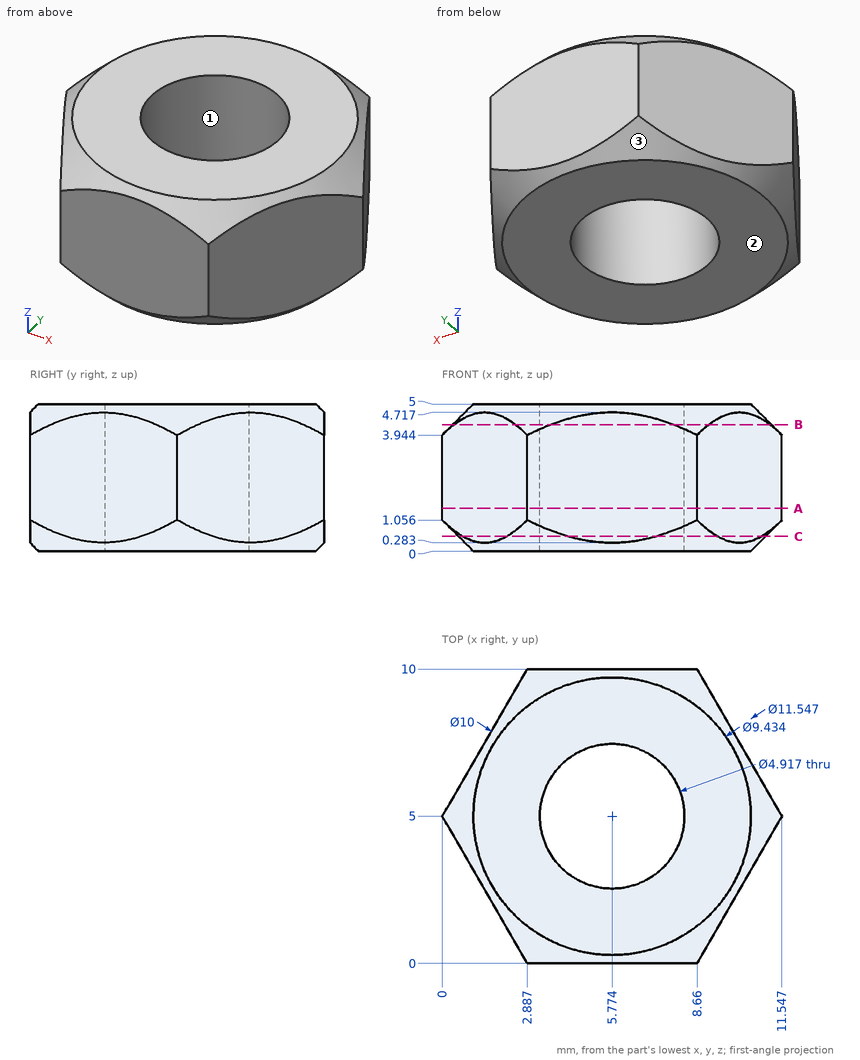
Verification items for this drawing (mm, ordinates from the low corner). Give positions to 0.01 mm unless a question says otherwise; leave off trailing zeros. Write each loop counter-clockwise with the first axis right and the second up, starting at its lowest first coordinate (ties: lowest second). Pieces come first, ordered by that corner, then holes.
1) Section check A-A, the plane z = 1.45. Record the boundary of the cut face in (x, y).
2) Section check B-B, the plane z = 4.3. Record the boundary of the cut face in (x, y) (1 decimal).
3) Section check C-C, the plane z = 0.5. Record the boundary of the cut face in (x, y) (1 decimal).
4) Material ranges on L1, parallel to Y at x = 8, z = 0.55 (1 decimal); L2, parallel to Y at x = 5.25, z = 2.7; L3, parallel to X at y = 1.5, z = 3.25 (1 decimal), recorded low to high.
5) Gauge pin test, flat ends, axial feed: pin 1 (3 mm diameter, centred on y = 1.5, z = 2.5, fed in from +X); pin 2 (2 mm diameter, centred on x = 7, y = 4.5, fed in from -Z). Record the tip position at first contact, or that the pin passes through.
6) Release check for a two-part mould opening along Y. For the marked faces 1, 2 and 3 record: pulls with the +Y half, pulls with the -Y half, needs draft (parallel to the pull), parting line crosses it, or undercut.
Computed:
1. outline: (0, 5) - (2.89, 0) - (8.66, 0) - (11.55, 5) - (8.66, 10) - (2.89, 10) - close; hole circle Ø4.92 at (5.77, 5)
2. outline: (0.4, 4.3) - (2.5, 0.7) arc R5.4 ccw to (3.7, 0) - (7.9, 0) arc R5.4 ccw to (9.1, 0.7) - (11.1, 4.3) arc R5.4 ccw to (11.1, 5.7) - (9.1, 9.3) arc R5.4 ccw to (7.9, 10) - (3.7, 10) arc R5.4 ccw to (2.5, 9.3) - (0.4, 5.7) arc R5.4 ccw to start; hole circle Ø4.9 at (5.8, 5)
3. outline: (0.7, 3.8) - (2.2, 1.2) arc R5.2 ccw to (4.3, 0) - (7.3, 0) arc R5.2 ccw to (9.4, 1.2) - (10.8, 3.8) arc R5.2 ccw to (10.8, 6.2) - (9.4, 8.8) arc R5.2 ccw to (7.3, 10) - (4.3, 10) arc R5.2 ccw to (2.2, 8.8) - (0.7, 6.2) arc R5.2 ccw to start; hole circle Ø4.9 at (5.8, 5)
4. L1: y = 0.2 to 4, 6 to 9.8
4. L2: y = 0 to 2.6, 7.4 to 10
4. L3: x = 2 to 9.5
5. pin 1: stops at x = 10.39
5. pin 2: passes through
6. face 1: undercut
6. face 2: needs draft
6. face 3: parting line crosses it
